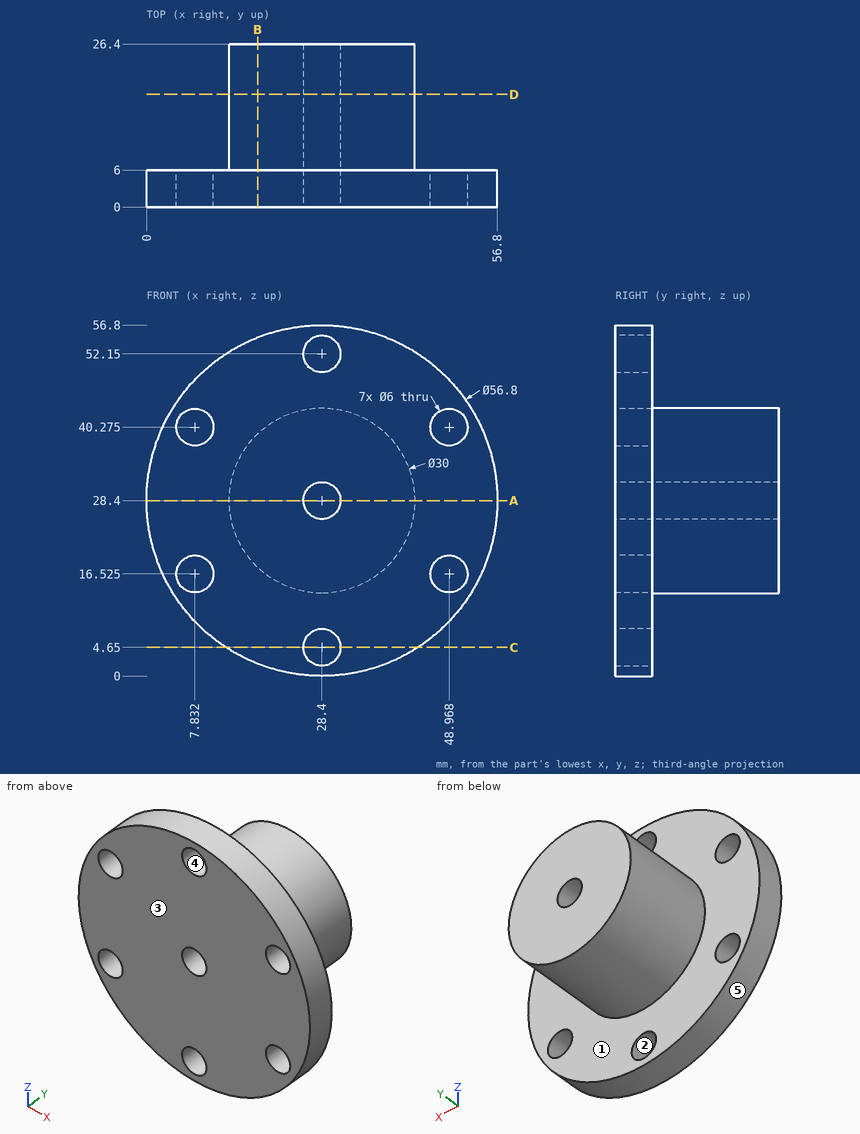
Job drawing, mm, ordinate dimensions from the low corner. One solid piece. A direction names the side the tool comes from. Give positions to 0.01 mm unless a question says otherwise; leave off trailing zeros. Order: outer loops, then holes, each group sorted by start corner. A loop starts at its lowest first (then second) coordinate and runs counter-clockwise, first axis right, second up. Notation, with made-up numbers: (66, -23.5) - (117, -23.5) arc R31 cw to (117, 8.5) - close; hole circle Ø1 at (65, 70). An arc over 180 degrees is marked (long way). Return JSON: item names as keys, results as strings.
1) Cut at D-D, the plane y = 18.25. Give the cut face in (x, z).
Geometry says:
{"outline": "circle Ø30 at (28.4, 28.4); hole circle Ø6 at (28.4, 28.4)"}
2) Cut at C-C, the plane z = 4.65. Give the cut face in (x, y).
Geometry says:
{"outline": "(12.83, 0) - (25.4, 0) - (25.4, 6) - (12.83, 6) - close; (31.4, 0) - (43.97, 0) - (43.97, 6) - (31.4, 6) - close"}
3) Cut at A-A, the plane z = 28.4. Give the cut face in (x, y), plus the area to 3 significant figures.
Geometry says:
{"outline": "(0, 0) - (25.4, 0) - (25.4, 26.4) - (13.4, 26.4) - (13.4, 6) - (0, 6) - close; (31.4, 0) - (56.8, 0) - (56.8, 6) - (43.4, 6) - (43.4, 26.4) - (31.4, 26.4) - close", "area": "794 mm²"}
4) 3-axis set-ups, long thin cutter, end or side, ignore diameter. For the marked faces 1 and 2: which of +Z, -Z, +X, -X, +Y, -Y reach the whole face in a straight line?
Geometry says:
{"face 1": "+Y", "face 2": "+Y, -Y"}
5) Probe line 1 (Z direction, x = 28.5, y = 17); line 2 (Y direction, x = 44.5, z = 35.5); line 3 (X direction, y = 3.25, z = 51). List the from-to ranges inside material, lowest first. Write a range as from..to.
Geometry says:
{"line 1": "13.4..25.4, 31.4..43.4", "line 2": "0..6", "line 3": "11.2..25.63, 31.17..45.6"}
6) Pull direction Z, two halves, no side cores. Call the marked faces 3, 4 and 5: pulls with the +Z half, pulls with the -Z half, needs draft (parallel to the pull), parting line crosses it, or undercut.
Geometry says:
{"face 3": "needs draft", "face 4": "undercut", "face 5": "parting line crosses it"}
7) Cut at B-B, the plane x = 18. Give the cut face in (y, z).
Geometry says:
{"outline": "(0, 1.97) - (6, 1.97) - (6, 17.59) - (26.4, 17.59) - (26.4, 39.21) - (6, 39.21) - (6, 54.83) - (0, 54.83) - close"}
8) Flat gauge pins, fed straight in: P1, Ø12, axis at y = 13, z = 33.5, coming from the +X side; P2, Ø3, axis at x = 29.5, y = 15, coming from the -Z side; P3, Ø10, axis at x = 50.5, y = 8.5, coming from the -Z side; P4, Ø3.5, axis at x = 48.97, z = 40.28, coming from the -Y side. Where does each tip first touch, or does it go through?
Geometry says:
{"P1": "x = 43.4", "P2": "z = 13.4", "P3": "z = 6.25", "P4": "through"}
